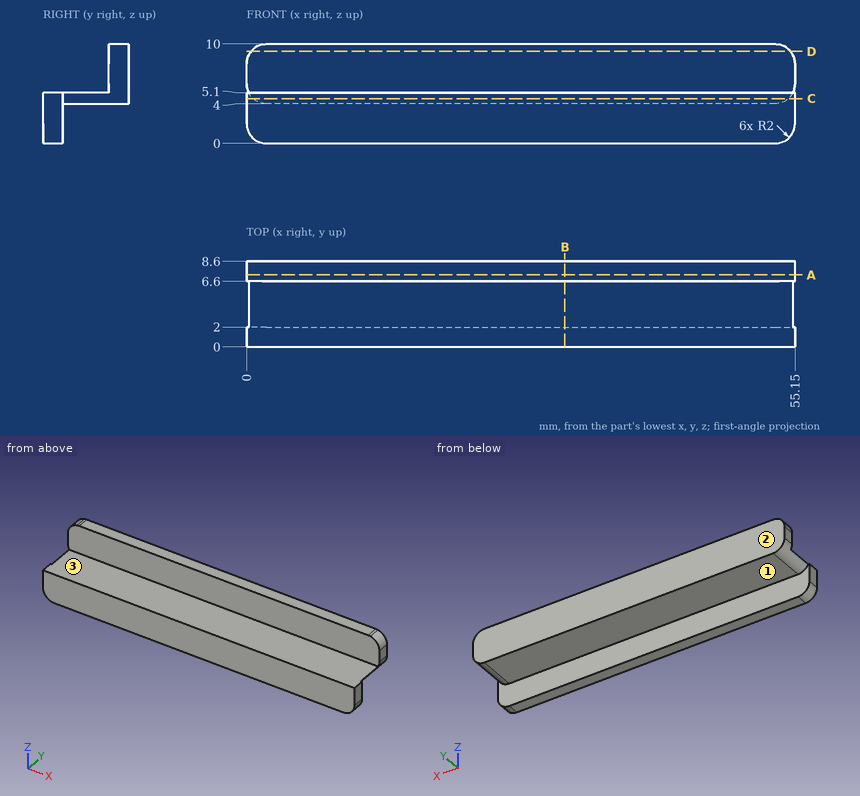
Geometry: see drawing. Coordinates: mm, zero at the bounding-box minimum. A direction names the side the tool comes from. Round coordinates to 2 decimals unless told otherwise and drop trailing zeros. Write each loop counter-clockwise with the first axis right and the second up, starting at its lowest first coordinate (ties: lowest second). Pieces come first, ordered by that corner, then holes. Notation, with made-up numbers: M 2.5,24 L 32.5,24 A9 ccw 32.5,34 Z; hole C 77.25,74 d4. An arc over 180 degrees is marked long. Answer in a Markdown table with one row per item. Add a question column.
(1) Contact query for flat-ended pins moving along their axis: pin 1 (5 mm diameter, centred on x = 36, y = 5.5, fed in from +Z); pin 2 (1.5 mm diameter, centred on x = 20, z = 1.5, fed in from +Y); pin 3 (2 mm diameter, centred on x = 21, y = 3.5, fed in from -Z); pin 4 (3.5 mm diameter, centred on x = 37, y = 2.5, fed in from +Z). Output: stop coordinate, or through.
(2) Ray query, L1, parallel to Z at x = 24, y = 7; L2, parallel to Z at x = 53, y = 3.5; L3, parallel to Y at x = 18, z = 7. Return the intervals inside material, ascending.
(3) Cut plane B-B, the plane x = 32. Return the cut outline in (y, z), then the cut area to 3 significant figures.
(4) Cut plane D-D, the plane z = 9.25. Return the cut outline in (x, y).
(5) Reachability of the marked faces 1, 2 and 3 from +Z, -Z, +X, -X, +Y, -Y: full face, straight path, thin tool, end or side. Return the list, or none.
(6) Cut plane C-C, the plane z = 4.5. Return the cut outline in (x, y).
(7) Cut plane A-A, the plane y = 7.25. Return the cut outline in (x, z).
Established:
| question | item | result |
|---|---|---|
| 1 | pin 1 | z = 10 |
| 1 | pin 2 | y = 2 |
| 1 | pin 3 | z = 4 |
| 1 | pin 4 | z = 5.1 |
| 2 | L1 | 4 to 10 |
| 2 | L2 | 4 to 5.1 |
| 2 | L3 | 6.6 to 8.6 |
| 3 | outline | M 0,0 L 2,0 L 2,4 L 8.6,4 L 8.6,10 L 6.6,10 L 6.6,5.1 L 0,5.1 Z |
| 3 | area | 27.3 mm² |
| 4 | outline | M 0.44,6.6 L 54.71,6.6 L 54.71,8.6 L 0.44,8.6 Z |
| 5 | face 1 | -Z, +X, -X, +Y |
| 5 | face 2 | +Z, -Z, +X, -X, +Y |
| 5 | face 3 | +Z, +X, -X, -Y |
| 6 | outline | M 0,0 L 55.15,0 L 55.15,2 L 54.47,2 L 54.47,8.6 L 0.68,8.6 L 0.68,2 L 0,2 Z |
| 7 | outline | M 0,6 A2 ccw 2,4 L 53.15,4 A2 ccw 55.15,6 L 55.15,8 A2 ccw 53.15,10 L 2,10 A2 ccw 0,8 Z |
